Source: CAD feature listing. Evaluate the final solid. Frame: model axes, mm. Coordinates: 2 decimals unless noted, no trailing zeros. Loops run counter-clockwise (first coordinate to the right, second up) from the corner with the lowest first, then second, coordinate; pieces in that order, holes last. Notation, with made-up numbers: M 47.5,6.5 L 70.5,6.5 A20 cw 70.5,40.5 Z; hole C -11.75,8 d5. An arc over 180 degrees is marked long. One line per question, with ' | ' between items. Start each with the question number.
1. Section query B-B, the plane z = 2.7. Output: boundary loops of the cut face in (x, y).
2. Section query D-D, the plane x = -7.5. Output: boundary loops of the cut face in (y, z).
3. Pin query (flat end, axial travel): P1, Ø1, axis at x = -7, z = 3.5, coming from the -Y side; P2, Ø2, axis at y = -1.5, z = 0.5, coming from the +X side. Return the tip coordinate at first contact, or that it passes through.
4. Ray query, probe 1 along Y at (x, z) = (0, 3.75); probe 2 along X at (y, z) = (-0.25, 0.85); probe 3 along X at (y, z) = (-2.5, 3.7). Return the intervals inside material, ascending.
5. Section query A-A, the plane x = 0. Output: boundary loops of the cut face in (y, z).
6. Mould query, pull axis X, two halves, no side actions, for faces 1 (the flat face through (2, 5, 0)), 2 (the cylindrical face through (-1.08, 4.88, 1.97)), 3 (the flat face through (6.526, -3.698, 1.972)). Classes: pulls with the +X half, pulls with the -X half, needs draft (parallel to the pull), parting line crosses it, or undercut.
7. Section query C-C, the plane y = 3.5. Output: boundary loops of the cut face in (x, z).
Autodesk Inventor part; units mm, degrees
ref_plane "YZ Plane" through (0, 0, 0) normal (1, 0, 0) x (0, 1, 0)
ref_plane "XZ Plane" through (0, 0, 0) normal (0, 1, 0) x (-1, 0, 0)
ref_plane "XY Plane" through (0, 0, 0) normal (0, 0, 1) x (1, 0, 0)
sketch "草图1" plane through (0, 0, 0) normal (0, 0, 1) x (1, 0, 0)
  circle A0 centre (0, 0) radius 5
  line L0 (4.3301, -7.5) -> (-4.3301, -7.5)
  line L1 (-4.3301, -7.5) -> (-8.6603, 0)
  line L2 (-8.6603, 0) -> (-4.3301, 7.5)
  line L3 (-4.3301, 7.5) -> (4.3301, 7.5)
  line L4 (4.3301, 7.5) -> (8.6603, 0)
  line L5 (8.6603, 0) -> (4.3301, -7.5)
  line L6 (0, 0) -> (0, 7.5)
  dimension "d0" = 10
  dimension "d1" = 15
extrude "拉伸1" add sketch "草图1" along normal blind 4
thread "螺纹1"
properties part number "刀轴带动盘连杆销螺帽"
Taken from the geometry:
1) outline: M -8.66,0 L -4.33,-7.5 L 4.33,-7.5 L 8.66,0 L 4.33,7.5 L -4.33,7.5 Z; hole C 0,0 d10
2) outline: M -2.01,0 L 2.01,0 L 2.01,4 L -2.01,4 Z
3) P1: y = -3.74 | P2: x = 8.37
4) probe 1: -7.5 to -5, 5 to 7.5 | probe 2: -8.52 to -4.99, 4.99 to 8.52 | probe 3: -7.22 to -4.33, 4.33 to 7.22
5) outline: M -7.5,0 L -5,0 L -5,4 L -7.5,4 Z; M 5,0 L 7.5,0 L 7.5,4 L 5,4 Z
6) face 1: needs draft | face 2: undercut | face 3: pulls with the +X half
7) outline: M -6.64,0 L -3.57,0 L -3.57,4 L -6.64,4 Z; M 3.57,0 L 6.64,0 L 6.64,4 L 3.57,4 Z
